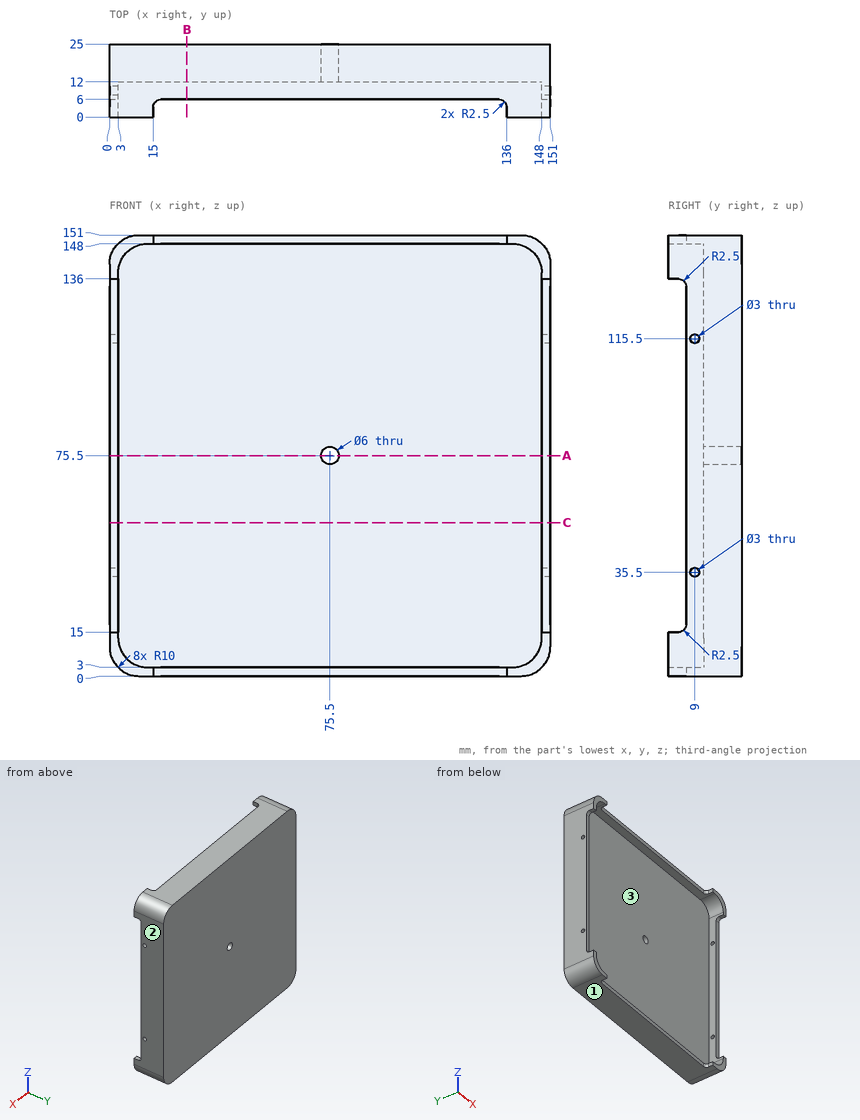
Here's the drawing with two shaded views (mm, measured from the low corner). I have some questions. Coordinates: 2 decimals unless noted, no trailing zeros. Write each loop counter-clockwise with the first axis right and the second up, starting at its lowest first coordinate (ties: lowest second). Pieces come first, ordered by that corner, then holes.
Item 1: I want a section at A-A on z = 75.5. Write out the boundary of the cut face in (x, y).
Item 2: If we mould it in two halves opening along Z, with no side actions, what happens to the marked faces 1, 2 and 3? For each: +Z half, -Z half, draft (parallel to the pull), parting line (faces both ways), or undercut.
Item 3: Will these pins go through, and if not, where does the flat tip stop? pin 1 (3.5 mm diameter, centred on y = 1.5, z = 1.5, fed in from +X); pin 2 (0.9 mm diameter, centred on x = 2, y = 2, fed in from -Z); pin 3 (2.5 mm diameter, centred on y = 1, z = 150, fed in from -X).
Item 4: I want a section at B-B on x = 26.5. Write out the boundary of the cut face in (y, z), and give its area (3 significant figures).
Item 5: If I drill on line 1 (Z direction, x = 71.5, y = 9.75); line 2 (Y direction, x = 1.05, z = 115.5), over which ranges is the centre line in solid material (lowest first)?
Item 6: I want a section at C-C on z = 52.5. Write out the boundary of the cut face in (x, y), and give its area (3 significant figures).
Findings below:
1. outline: (0, 6) - (3, 6) - (3, 12) - (72.5, 12) - (72.5, 25) - (0, 25) - close; (78.5, 12) - (148, 12) - (148, 6) - (151, 6) - (151, 25) - (78.5, 25) - close
2. face 1: -Z half
2. face 2: draft
2. face 3: undercut
3. pin 1: stops at x = 148.38
3. pin 2: stops at z = 3.44
3. pin 3: stops at x = 3.68
4. outline: (6, 0) - (25, 0) - (25, 151) - (6, 151) - (6, 148) - (12, 148) - (12, 3) - (6, 3) - close
4. area: 2,000 mm2
5. line 1: z = 0 to 3, 148 to 151
5. line 2: y = 6 to 7.5, 10.5 to 25
6. outline: (0, 6) - (3, 6) - (3, 12) - (148, 12) - (148, 6) - (151, 6) - (151, 25) - (0, 25) - close
6. area: 2,000 mm2
